Job drawing, mm, ordinate dimensions from the low corner. One solid piece. A direction names the side the tool comes from. Give positions to 0.01 mm unless a question says otherwise; leave off trailing zeros. Order: outer loops, then holes, each group sorted by start corner. A loop starts at its lowest first (then second) coordinate and runs counter-clockwise, first axis right, second up.
1. Slice it at C-C on x = 21. List the corners of the cut face in (y, z), and give its area (3 significant figures).
2. Drop flat-ended pins along their axis: pin 1 Ø2 at (x, z) = (19.5, 4.5) entering from -Y; pin 2 Ø1.6 at (y, z) = (36, 3.5) entering from -X. Give the stop position or say it passes through.
3. Probe line 1 (X direction, y = 15, z = 2); line 2 (Z direction, x = 10.25, y = 34.5); line 3 (Y direction, x = 20.25, z = 1.5). List the from-to ranges inside material, lowest first.
4. Which spindle directions (+Z, -Z, +X, -X, +Y, -Y) get a long thin tool onto all of the face, cutting with end or side? Do the marked faces 1 and 2. Say none if no direction does.
5. Slice it at A-A on z = 1.75. List the corners of the cut face in (x, y), and give its area (3 significant figures).
6. Slice it at B-B on y = 13.5. List the corners of the cut face in (x, z), and give its area (4 significant figures).
7. Slice it at D-D on x = 13.75. List the corners of the cut face in (y, z).
8. Mould opens along X. For the marked faces 3, 4, 5 and 6 say: +X half, -X half, draft (parallel to the pull), parting line (faces both ways), or undercut.
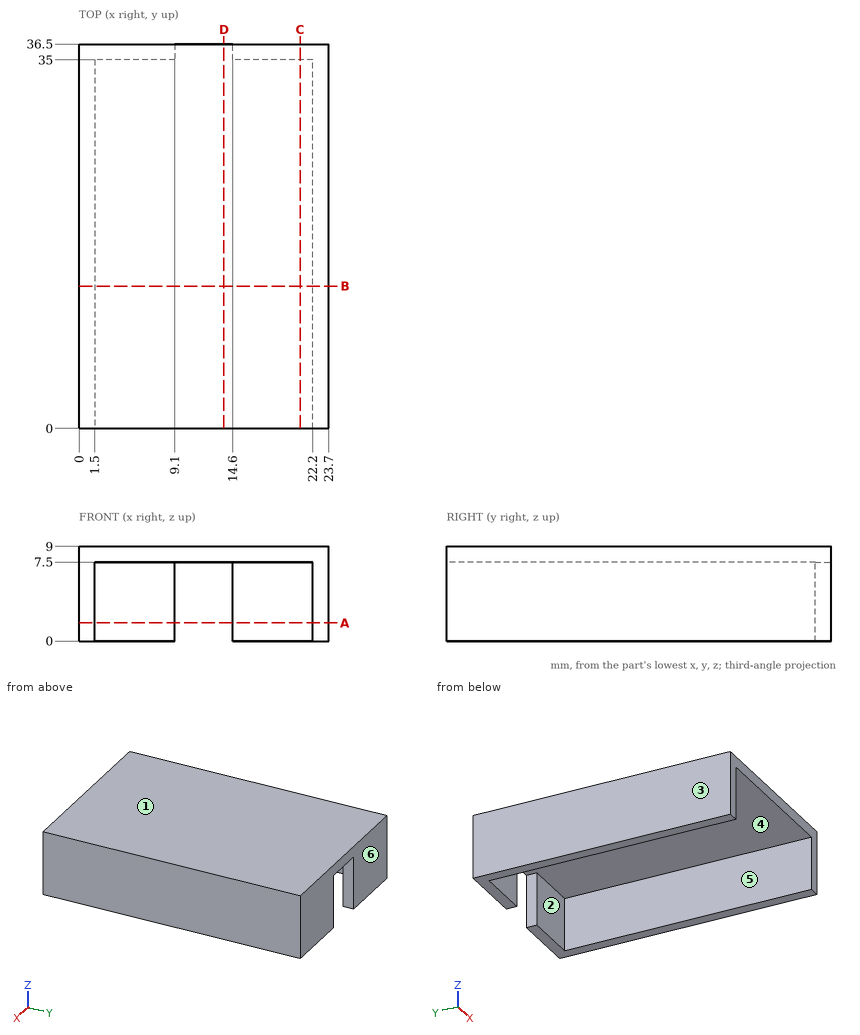
Data:
1. outline: (0, 7.5) - (35, 7.5) - (35, 0) - (36.5, 0) - (36.5, 9) - (0, 9) - close
1. area: 66.0 mm2
2. pin 1: stops at y = 35
2. pin 2: stops at x = 0
3. line 1: x = 0 to 1.5, 22.2 to 23.7
3. line 2: z = 7.5 to 9
3. line 3: y = 35 to 36.5
4. face 1: +Z, +X, -X, +Y, -Y
4. face 2: -Z, -Y
5. outline: (0, 0) - (1.5, 0) - (1.5, 35) - (9.1, 35) - (9.1, 36.5) - (0, 36.5) - close; (14.6, 35) - (22.2, 35) - (22.2, 0) - (23.7, 0) - (23.7, 36.5) - (14.6, 36.5) - close
5. area: 132 mm2
6. outline: (0, 0) - (1.5, 0) - (1.5, 7.5) - (22.2, 7.5) - (22.2, 0) - (23.7, 0) - (23.7, 9) - (0, 9) - close
6. area: 58.05 mm2
7. outline: (0, 7.5) - (36.5, 7.5) - (36.5, 9) - (0, 9) - close
8. face 3: -X half
8. face 4: undercut
8. face 5: undercut
8. face 6: draft
